The drawing under review shows one solid part. Ordinate dimensions are in mm from its lowest x, y, z. Give positions to 0.01 mm unless a question says otherwise; leave off trailing zeros. Loops run counter-clockwise (first coordinate to the right, second up) from the corner with the lowest first, then second, coordinate; pieces in that order, holes last. Notation, with made-up numbers: M -16,59.25 L 38,59.25 A19 ccw 38,74.25 Z; hole C 37,40.5 d1. An arc over 180 degrees is marked long. Write item = value, one per line. Start each with the question number.
1. We need section A-A on z = 15. Give the boundary of the cut face in (x, y), then the cut area to 3 significant figures.
2. We need section C-C on y = 4.5. Count the separate pieces of the cut face and the enclosed holes in it, then the cut area to 3 significant figures.
3. We need section B-B on x = 15. Give the boundary of the cut face in (y, z).
4. We need section D-D on z = 10.25. Give the boundary of the cut face in (x, y).
5. Wall thickness on line 1 along X through (y, z) = (2.5, 15); line 2 along Z through (x, y) = (14, 5.5) (1 decimal); line 3 along Z through (x, y) = (26.5, 5.25) (1 decimal): over which ranges is each line inside the solid? List them lowest first. Write a range as from..to.
6. For pin 1 (5 mm diameter, centred on x = 15, z = 15, fed in from -Y), flat-tipped, find the tip position at first contact; note if it passes through.
7. Draft analysis for pull direction X (two halves, no side actions). For the marked faces 1, 2 and 3, state which applies: pulls with the +X half, pulls with the -X half, needs draft (parallel to the pull), parting line crosses it, or undercut.
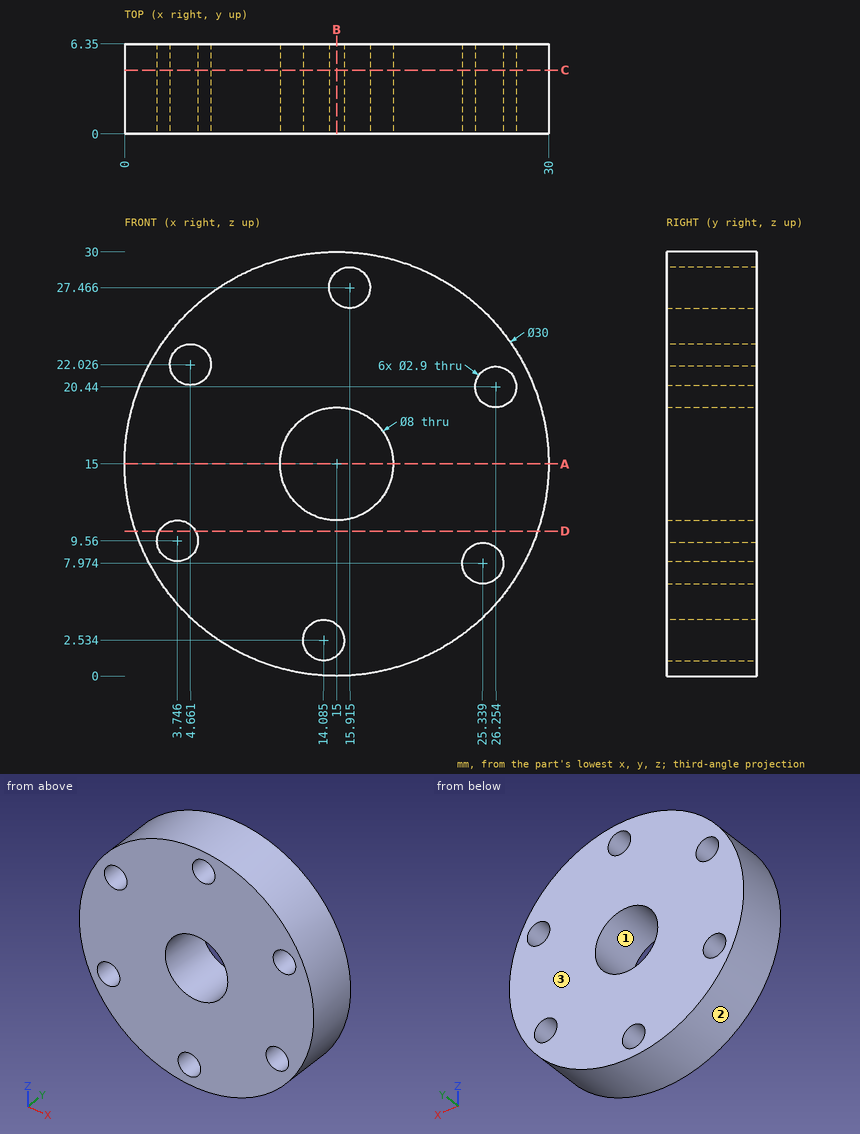
Final values:
q1.outline = M 0,0 L 11,0 L 11,6.35 L 0,6.35 Z; M 19,0 L 30,0 L 30,6.35 L 19,6.35 Z
q1.area = 140 mm²
q2.separate_pieces = 1
q2.enclosed_holes = 7
q2.area = 617 mm²
q3.outline = M 0,0 L 6.35,0 L 6.35,1.41 L 0,1.41 Z; M 0,3.66 L 6.35,3.66 L 6.35,11 L 0,11 Z; M 0,19 L 6.35,19 L 6.35,26.34 L 0,26.34 Z; M 0,28.59 L 6.35,28.59 L 6.35,30 L 0,30 Z
q4.outline = M 0.77,0 L 2.47,0 L 2.47,6.35 L 0.77,6.35 Z; M 5.02,0 L 29.23,0 L 29.23,6.35 L 5.02,6.35 Z
q5.line_1 = 0..11, 19..30
q5.line_2 = 0..1.1, 4..11.1, 18.9..30
q5.line_3 = 5.4..7.1, 8.8..19, 21.9..24.6
q6.pin_1 = through
q7.face_1 = undercut
q7.face_2 = parting line crosses it
q7.face_3 = needs draft
